from build123d import *

# Parameters (mm, degrees)
BOSS_EXTRUDE1_DEPTH                            = 6.35
CSK_FOR_4_FLAT_HEAD_MACHINE_SCREW1_D           = 3.2639
CSK_FOR_4_FLAT_HEAD_MACHINE_SCREW1_CSINK_D     = 5.715
CSK_FOR_4_FLAT_HEAD_MACHINE_SCREW1_CSINK_ANGLE = 82


with BuildPart() as part:
    # Sketch1 → Boss-Extrude1 (new body)
    with BuildSketch(Plane(origin=(0, 0, 0), x_dir=(0, 0, -1), z_dir=(1, 0, 0))):
        Polygon((0, 0), (76.2, 131.982271537), (119.58608314, 131.982271537), (195.78608314, 0), (151.791992628, 0), (97.89304157, 93.355721707), (43.994090512, 0), align=None)
    extrude(amount=BOSS_EXTRUDE1_DEPTH)

    # CSK for #4 Flat Head Machine Screw1 (through all)
    with Locations(Plane.ZY):
        with Locations((-161.066379527, 12.511290682), (-138.841379527, 51.00611988), (-56.944703613, 51.00611988), (-34.719703613, 12.511290682)):
            CounterSinkHole(CSK_FOR_4_FLAT_HEAD_MACHINE_SCREW1_D / 2, CSK_FOR_4_FLAT_HEAD_MACHINE_SCREW1_CSINK_D / 2, counter_sink_angle=CSK_FOR_4_FLAT_HEAD_MACHINE_SCREW1_CSINK_ANGLE)


solid = part.part
Part model, mm, in its own coordinate system. Round coordinates to 2 decimals unless told otherwise and drop trailing zeros. Write each loop counter-clockwise with the first axis right and the second up, starting at its lowest first coordinate (ties: lowest second). Pieces come first, ordered by that corner, then holes. Notation, with made-up numbers: (32.5, 31) - (69.5, 31) arc R13 ccw to (69.5, 46) - close; hole circle Ø3 at (75, 55.25). An arc over 180 degrees is marked (long way). Use CSV: the item, a comma, the result in double quotes.
Item 1: Flat gauge pins, fed straight in: P1, Ø3, axis at y = 12.51, z = -161.07, coming from the -X side; P2, Ø5, axis at y = 51.01, z = -56.94, coming from the -X side; P3, Ø1, axis at x = 1, y = 69.5, coming from the -Z side; P4, Ø2, axis at x = 5, y = 44, coming from the -Z side. Where does each tip first touch, or does it go through?
Results list:
P1,"passes through"
P2,"stops at x = 0.4"
P3,"stops at z = -155.95"
P4,"stops at z = -170.96"
Item 2: Slice it at C-C, the plane z = -24. Write the cut outline in (x, y), then the cut area to 3 significant figures.
Results list:
outline,"(0, 0) - (6.35, 0) - (6.35, 41.57) - (0, 41.57) - close"
area,"264 mm²"
Item 3: Slice it at D-D, the plane y = 103. Write the cut outline in (x, z).
Results list:
outline,"(0, -136.32) - (6.35, -136.32) - (6.35, -59.47) - (0, -59.47) - close"
Item 4: Wall check: L1, parallel to Z at x = 3.5, y = 20.5; L2, parallel to Z at x = 2, y = 13.5; L3, parallel to Z at x = 4.5, y = 9. Give the ranges that are in metal, low to high.
Results list:
L1,"z = -183.95 to -139.96, -55.83 to -11.84"
L2,"z = -187.99 to -162.36, -159.77 to -144, -51.79 to -36.02, -33.42 to -7.79"
L3,"z = -190.59 to -146.6, -49.19 to -5.2"
Item 5: Pull direction Z, two halves, no side cores. Call faces 1 (the flat face through (3, 131.982, -98)), 2 (the flat face through (3.13, 65.07, -37.57)), 3 (the flat face through (3.131, 46.024, -125.22)), 4 (the flat face through (3.13, 47.33, -71.32)): pulls with the +Z half, pulls with the -Z half, needs draft (parallel to the pull), parting line crosses it, or undercut.
Results list:
face 1,"needs draft"
face 2,"pulls with the +Z half"
face 3,"undercut"
face 4,"undercut"
Item 6: Slice it at B-B, the plane x = 3.5. Write the cut outline in (y, z), then the cut area to 3 significant figures.
Results list:
outline,"(0, -195.79) - (131.98, -119.59) - (131.98, -76.2) - (0, 0) - (0, -43.99) - (93.36, -97.89) - (0, -151.79) - close; hole circle Ø3.26 at (12.51, -161.07); hole circle Ø3.26 at (12.51, -34.72); hole circle Ø3.26 at (51.01, -138.84); hole circle Ø3.26 at (51.01, -56.94)"
area,"10,700 mm²"
Item 7: Slice it at A-A, the plane y = 66. Write the cut outline in (x, z), then the cut area to 3 significant figures.
Results list:
outline,"(0, -157.68) - (6.35, -157.68) - (6.35, -113.69) - (0, -113.69) - close; (0, -82.1) - (6.35, -82.1) - (6.35, -38.11) - (0, -38.11) - close"
area,"559 mm²"
